```python
from build123d import *

# Parameters (mm, degrees)
BOSS_EXTRUDE1_DEPTH   = 5.08
M2X0_4_TAPPED_HOLE1_D = 1.6
SKETCH8_W             = 12.065
SKETCH8_H             = 9.8933
BOSS_EXTRUDE2_DEPTH   = 19.8628
FILLET1_R             = 1.27
FILLET2_R             = 0.635
FILLET3_R             = 0.635
SKETCH9_W             = 9.0551
SKETCH9_H             = 4.5085
BOSS_EXTRUDE3_DEPTH   = 1.0795


with BuildPart() as part:
    # Sketch1 → Boss-Extrude1 (new body)
    with BuildSketch(Plane(origin=(0, 0, 0), x_dir=(1, 0, 0), z_dir=(0, 1, 0))):
        with BuildLine():
            Line((8.46455, -4.0132), (-8.46455, -4.0132))
            ThreePointArc((-8.46455, -4.0132), (-12.47775, 0), (-8.46455, 4.0132))
            Line((-8.46455, 4.0132), (8.46455, 4.0132))
            ThreePointArc((8.46455, 4.0132), (12.47775, 0), (8.46455, -4.0132))
        make_face()
    extrude(amount=BOSS_EXTRUDE1_DEPTH)

    # M2x0.4 Tapped Hole1 (through all)
    with Locations(Plane(origin=(0, 5.08, 0), x_dir=(1, 0, 0), z_dir=(0, 1, 0))):
        with Locations((-8.46455, 0), (8.46455, 0)):
            Hole(M2X0_4_TAPPED_HOLE1_D / 2)

    # Sketch8 → Boss-Extrude2 (add)
    with BuildSketch(Plane(origin=(0, 5.08, 0), x_dir=(1, 0, 0), z_dir=(0, 1, 0))):
        Rectangle(SKETCH8_W, SKETCH8_H)
    extrude(amount=-BOSS_EXTRUDE2_DEPTH)

    # Fillet1
    fillet1_edges = [part.edges().sort_by_distance(p)[0] for p in [
        (-6.0325, -4.8514, 4.94665),
        (6.0325, -4.8514, 4.94665),
        (-6.0325, -4.8514, -4.94665),
        (6.0325, -4.8514, -4.94665),
    ]]
    fillet(fillet1_edges, radius=FILLET1_R)

    # Fillet2
    fillet2_edges = [part.edges().sort_by_distance(p)[0] for p in [
        (-7.225822742, 0, 4.0132),
        (-12.47775, 0, 0),
        (-7.225822742, 0, -4.0132),
        (7.225822742, 0, -4.0132),
        (7.225822742, 0, 4.0132),
        (12.47775, 0, 0),
    ]]
    fillet(fillet2_edges, radius=FILLET2_R)

    # Fillet3
    fillet3_edges = [part.edges().sort_by_distance(p)[0] for p in [
        (-6.0325, -14.7828, 0),
        (0, -14.7828, 4.94665),
        (0, -14.7828, -4.94665),
        (6.0325, -14.7828, 0),
        (5.660525612, -14.7828, -4.574675612),
        (-5.660525612, -14.7828, -4.574675612),
        (5.660525612, -14.7828, 4.574675612),
        (-5.660525612, -14.7828, 4.574675612),
    ]]
    fillet(fillet3_edges, radius=FILLET3_R)

    # Sketch9 → Boss-Extrude3 (add)
    with BuildSketch(Plane(origin=(0, 5.08, 0), x_dir=(1, 0, 0), z_dir=(0, 1, 0))):
        Rectangle(SKETCH9_W, SKETCH9_H)
    extrude(amount=BOSS_EXTRUDE3_DEPTH)


solid = part.part
```
Could you check a few things on this model? Use its own coordinates, in mm. A direction names the side the tool comes from. Coordinates: 2 decimals unless noted, no trailing zeros. Write each loop counter-clockwise with the first axis right and the second up, starting at its lowest first coordinate (ties: lowest second). Pieces come first, ordered by that corner, then holes. Notation, with made-up numbers: (43, -14.75) -> (66, -14.75) arc R29 cw to (66, 11.25) -> close; hole circle Ø7 at (34.5, 67.25). An arc over 180 degrees is marked (long way). One line per question, with ' | ' between items. Start each with the question number.
1. If we section it at C-C (y = -3): Please give me the cut outline in (x, z), and give its area (3 significant figures).
2. Thinking about a two-plate mould opening in X: for faces 1 (the face through (0, -4, -4.947)), 2 (the face through (-5.67, -4.668, -4.565)), 3 (the face through (9.264, 2.504, -0.035)), which applies, pulls with the +X half, pulls with the -X half, needs draft (parallel to the pull), parting line crosses it, or undercut?
3. If we section it at B-B (y = 1.5): Please give me the cut outline in (x, z).
4. For faces 4 (the face through (7, 3, 4.013)), 5 (the face through (-5.67, -4.668, 4.565)), 6 (the face through (7, 3, -4.013)), which set-ups out of +Z, -Z, +X, -X, +Y, -Y let a thin tool reach every point of the face, with its end or its side?
5. Please list where these lines run through material, in increasing order: line 1 along X through (y, z) = (0.5, -0.25); line 2 along Y through (x, z) = (-7, 1.25); line 3 along X through (y, z) = (-10.5, -3).
6. If we section it at D-D (x = 7): Please give me the cut outline in (y, z) (3 decimals).
7. If we section it at A-A (z = 0): Please give me the cut outline in (x, y) (1 decimal), and give its area (3 significant figures).
8. Will these pins go through, and if not, where does the flat tip stop? P1, Ø0.7, axis at x = -7, y = 2, coming from the +Z side; P2, Ø2.5, axis at x = 7, y = 2, coming from the -Z side; P3, Ø2, axis at x = -8.46, z = 0, coming from the +Y side; P4, Ø2, axis at x = -5.5, z = 1, coming from the -Y side.
Return value:
1) outline: (-6.03, -3.68) arc R1.27 ccw to (-4.76, -4.95) -> (4.76, -4.95) arc R1.27 ccw to (6.03, -3.68) -> (6.03, 3.68) arc R1.27 ccw to (4.76, 4.95) -> (-4.76, 4.95) arc R1.27 ccw to (-6.03, 3.68) -> close | area: 118 mm²
2) face 1: needs draft | face 2: pulls with the -X half | face 3: undercut
3) outline: (-8.46, -4.01) -> (-5.99, -4.01) arc R1.27 ccw to (-4.76, -4.95) -> (4.76, -4.95) arc R1.27 ccw to (5.99, -4.01) -> (8.46, -4.01) arc R4.01 ccw to (8.46, 4.01) -> (5.99, 4.01) arc R1.27 ccw to (4.76, 4.95) -> (-4.76, 4.95) arc R1.27 ccw to (-5.99, 4.01) -> (-8.46, 4.01) arc R4.01 ccw to start; hole circle Ø1.6 at (-8.46, 0); hole circle Ø1.6 at (8.46, 0)
4) face 4: +Z, +X, +Y, -Y | face 5: +Z, -X, -Y | face 6: -Z, +X, +Y, -Y
5) line 1: x = -12.46 to -9.22, -7.7 to 7.7, 9.22 to 12.46 | line 2: y = 0 to 5.08 | line 3: x = -6.03 to 6.03
6) outline: (0, -3.378) arc R0.635 ccw to (0.635, -4.013) -> (5.08, -4.013) -> (5.08, 4.013) -> (0.635, 4.013) arc R0.635 ccw to (0, 3.378) -> close
7) outline: (-12.5, 0.6) arc R0.6 ccw to (-11.8, 0) -> (-9.3, 0) -> (-9.3, 5.1) -> (-12.5, 5.1) -> close; (-7.7, 0) -> (-6, 0) -> (-6, -14.1) arc R0.6 ccw to (-5.4, -14.8) -> (5.4, -14.8) arc R0.6 ccw to (6, -14.1) -> (6, 0) -> (7.7, 0) -> (7.7, 5.1) -> (4.5, 5.1) -> (4.5, 6.2) -> (-4.5, 6.2) -> (-4.5, 5.1) -> (-7.7, 5.1) -> close; (9.3, 0) -> (11.8, 0) arc R0.6 ccw to (12.5, 0.6) -> (12.5, 5.1) -> (9.3, 5.1) -> close | area: 298 mm²
8) P1: stops at z = 4.01 | P2: stops at z = -4.48 | P3: stops at y = 5.08 | P4: stops at y = -14.78
